Check sheet for the modelled part. Datum: model origin and axes. Units: mm. Face numbers are marked on the shaded views. Round coordinates to 2 decimals unless told otherwise and drop trailing zeros. Loops run counter-clockwise (first coordinate to the right, second up) from the corner with the lowest first, then second, coordinate; pieces in that order, holes last. Notation, with made-up numbers: (78.5, 82) -> (116.5, 82) arc R19 ccw to (116.5, 99) -> close; hole circle Ø10 at (-8, -30.5). An arc over 180 degrees is marked (long way). Return JSON: item names as keys, results as strings.
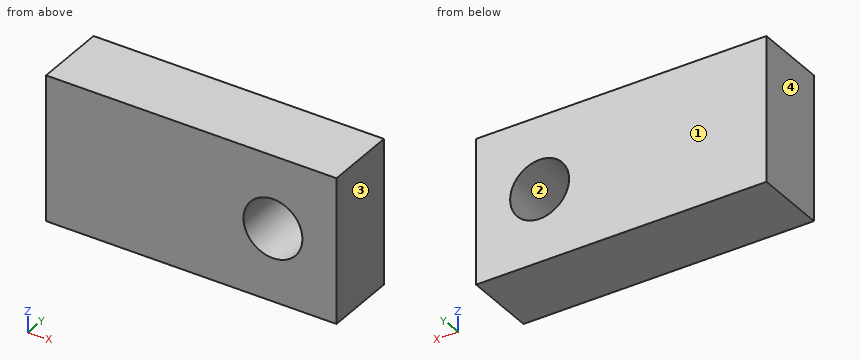
from build123d import *

# Parameters (mm, degrees)
F0_W     = 50.8
F0_H     = 25.4
F0_R     = 5.1562
F1_DEPTH = 6.35


with BuildPart() as f1:
    # F0 (on Front) → F1 (new body, symmetric)
    with BuildSketch(Plane.XZ):
        Rectangle(F0_W, F0_H)
        with Locations((14.2875, 0)):
            Circle(F0_R, mode=Mode.SUBTRACT)
    extrude(amount=F1_DEPTH, both=True)


solid = f1.part
Q1. Material ranges on line 1 (Z direction, x = 14, y = 4.25); line 2 (X direction, y = -5.25, z = -4.25); line 3 (Z direction, x = 11.5, y = -2.25), recorded low to high.
Results list:
{"line 1": "-12.7 to -5.15, 5.15 to 12.7", "line 2": "-25.4 to 11.37, 17.21 to 25.4", "line 3": "-12.7 to -4.34, 4.34 to 12.7"}
Q2. Draft check along X on the marked faces 1, 2, 3 and 4. Enter one of: released by +X, released by -X, zero draft, split by the parting line, or undercut.
Results list:
{"face 1": "zero draft", "face 2": "undercut", "face 3": "released by +X", "face 4": "released by -X"}
Q3. Go/stop test with a flat-tipped pin: pin 1 (6 mm diameter, centred on x = 14.29, z = 0, fed in from -Y). Record where the tip stops, or that it passes through.
Results list:
{"pin 1": "through"}
Q4. Section check B-B (y = 0). Record the boundary of the cut face in (x, z).
Results list:
{"outline": "(-25.4, -12.7) -> (25.4, -12.7) -> (25.4, 12.7) -> (-25.4, 12.7) -> close; hole circle Ø10.31 at (14.29, 0)"}
Q5. Section check C-C (z = -3). Record the boundary of the cut face in (x, y), then the cut area to 3 significant figures.
Results list:
{"outline": "(-25.4, -6.35) -> (10.09, -6.35) -> (10.09, 6.35) -> (-25.4, 6.35) -> close; (18.48, -6.35) -> (25.4, -6.35) -> (25.4, 6.35) -> (18.48, 6.35) -> close", "area": "539 mm^2"}
Q6. Section check A-A (z = 0). Record the boundary of the cut face in (x, y), then the cut area to 3 significant figures.
Results list:
{"outline": "(-25.4, -6.35) -> (9.13, -6.35) -> (9.13, 6.35) -> (-25.4, 6.35) -> close; (19.44, -6.35) -> (25.4, -6.35) -> (25.4, 6.35) -> (19.44, 6.35) -> close", "area": "514 mm^2"}
